from build123d import *

# Parameters (mm, degrees)
BOSS_EXTRUDE1_DEPTH     = 110
SKETCH2_R               = 8.1
CUT_EXTRUDE1_DEPTH      = 41
CUT_EXTRUDE2_DEPTH      = 74
CUT_EXTRUDE2_DEPTH_BACK = 41
SKETCH3_R               = 2.25
CUT_EXTRUDE3_DEPTH      = 21
SKETCH5_R               = 3.6
CUT_EXTRUDE4_DEPTH      = 17
SKETCH6_R               = 10
SKETCH6_R_2             = 2
CUT_EXTRUDE5_DEPTH      = 149
SKETCH7_R               = 1.5
CUT_EXTRUDE6_DEPTH      = 43


with BuildPart() as part:
    # Sketch1 → Boss-Extrude1 (new body)
    with BuildSketch(Plane.XY):
        with BuildLine():
            Line((0, 0), (40, 0))
            Line((40, 0), (20, -79.858784278))
            ThreePointArc((20, -79.858784278), (12.904134464, -90.766668728), (0.599169725, -95))
            Line((0.599169725, -95), (-73, -95))
            Line((-73, -95), (-73, -75))
            Line((-73, -75), (-20, -75))
            ThreePointArc((-20, -75), (-5.857864376, -69.142135624), (0, -55))
            Line((0, -55), (0, 0))
        make_face()
    extrude(amount=BOSS_EXTRUDE1_DEPTH)

    # Sketch2 → Cut-Extrude1 (cut, through all)
    with BuildSketch(Plane(origin=(0, -4.784896585, 0), x_dir=(0, 0, -1), z_dir=(1, 0, 0))):
        with Locations((-55, 4.784896585)):
            Circle(SKETCH2_R)
    extrude(amount=CUT_EXTRUDE1_DEPTH, mode=Mode.SUBTRACT)

    # Sketch4 → Cut-Extrude2 (cut, two sides)
    with BuildSketch(Plane.ZY) as cut_extrude2_sk:
        Polygon((33, 0), (0, -95), (0, 0), align=None)
        Polygon((77, 0), (110, -95), (110, 0), align=None)
    extrude(amount=CUT_EXTRUDE2_DEPTH, mode=Mode.SUBTRACT)
    extrude(cut_extrude2_sk.sketch, amount=-CUT_EXTRUDE2_DEPTH_BACK, mode=Mode.SUBTRACT)

    # Sketch3 → Cut-Extrude3 (cut, through all)
    with BuildSketch(Plane(origin=(0, -75, 0), x_dir=(1, 0, 0), z_dir=(0, 1, 0))):
        with Locations((-62.4, -12.5)):
            Circle(SKETCH3_R)
        with Locations((-62.4, -97.5)):
            Circle(SKETCH3_R)
        with Locations((-37.4, -12.5)):
            Circle(SKETCH3_R)
        with Locations((-37.4, -97.5)):
            Circle(SKETCH3_R)
    extrude(amount=-CUT_EXTRUDE3_DEPTH, mode=Mode.SUBTRACT)

    # Sketch5 → Cut-Extrude4 (cut)
    with BuildSketch(Plane(origin=(0, 0, 0), x_dir=(1, 0, 0), z_dir=(0, 1, 0))):
        with Locations((7, -40)):
            Circle(SKETCH5_R)
        with Locations((32, -40)):
            Circle(SKETCH5_R)
        with Locations((7, -70)):
            Circle(SKETCH5_R)
        with Locations((32, -70)):
            Circle(SKETCH5_R)
    extrude(amount=-CUT_EXTRUDE4_DEPTH, mode=Mode.SUBTRACT)

    # Sketch6 → Cut-Extrude5 (cut)
    with BuildSketch(Plane.ZY.offset(73)):
        with Locations((55, -95)):
            Circle(SKETCH6_R)
        with Locations((30, -85)):
            Circle(SKETCH6_R_2)
        with Locations((80, -85)):
            Circle(SKETCH6_R_2)
    extrude(amount=-CUT_EXTRUDE5_DEPTH, mode=Mode.SUBTRACT)

    # Sketch7 → Cut-Extrude6 (cut)
    with BuildSketch(Plane(origin=(37.639221534, -9.426444911, 0), x_dir=(0, 0, -1), z_dir=(0.970041514, -0.242939214, 0))):
        with Locations((-75, -22.607551707)):
            Circle(SKETCH7_R)
        with Locations((-35, -22.607551707)):
            Circle(SKETCH7_R)
    extrude(amount=-CUT_EXTRUDE6_DEPTH, mode=Mode.SUBTRACT)


solid = part.part
CAD build for the part. Positions are in the model's coordinates, mm. A direction names the side the tool comes from. Give positions to 0.01 mm unless a question says otherwise; leave off trailing zeros. Loops run counter-clockwise (first coordinate to the right, second up) from the corner with the lowest first, then second, coordinate; pieces in that order, holes last. Notation, with made-up numbers: M 79,-2 L 136,-2 A34 ccw 136,37 Z; hole C -30.75,33.5 d2. An arc over 180 degrees is marked long. Answer in a Markdown table with one row per item. Add a question column.
Item 1: Drop flat-ended pins along their axis: P1, Ø6, axis at x = -55, z = 86.5, coming from the +Y side; P2, Ø10, axis at y = -57.5, z = 14, coming from the +X side; P3, Ø6, axis at x = 32, z = 40, coming from the +Y side; P4, Ø7, axis at x = -37.4, z = 97.5, coming from the -Y side. Give the stop position or say it passes through.
Item 2: Band-saw the part on B-B on z = 30. Give the cut face in (x, y), then the cut area to 3 significant figures.
Item 3: Probe probe 1 along X at (y, z) = (-5, 70); probe 2 along Z at (x, y) = (-37.4, -82.5); probe 3 along Z at (x, y) = (-37.5, -80). List the from-to ranges inside material, lowest first.
Item 4: Band-saw the part on C-C on y = -14.5. Give the cut face in (x, z), then the cut area to 3 significant figures.
Item 5: Mould opens along Z. For faces 4 (the face through (-47, -75, 54)), 5 (the face through (7.82, -57.391, 96.936)), 6 (the face through (16.329, -26.35, 36.106)), 7 (the face through (-27.679, -83.314, 31.075)) say: +Z half, -Z half, draft (parallel to the pull), parting line (faces both ways), or undercut.
Item 6: Band-saw the part on A-A on x = -37.4. Give the cut face in (y, z).
Item 7: Band-saw the part on D-D on z = 70. Give the cut face in (x, y), then the cut area to 3 significant figures.
Item 8: Tool access for faces 1 (the face through (32, -17, 40)), 2 (the face through (0, -34, 54)), 3 (the face through (-36, -95, 22)): list every direction of +Z, -Z, +X, -X, +Y, -Y with a clear straight run to the whole face (end or side of a thin tool).
Reply:
| question | item | result |
|---|---|---|
| 1 | P1 | stops at y = -75 |
| 1 | P2 | stops at x = 26.84 |
| 1 | P3 | stops at y = -17 |
| 1 | P4 | stops at y = -95 |
| 2 | outline | M -73,-95 L 0.6,-95 A20 ccw 16.6,-87 L -73,-87 Z; M -73,-83 L 18.93,-83 A20 ccw 20,-79.86 L 37.84,-8.64 L 0,-8.64 L 0,-55 A20 cw -20,-75 L -73,-75 Z |
| 2 | area | 3,470 mm^2 |
| 3 | probe 1 | x = 0 to 3.4, 10.6 to 28.4, 35.6 to 38.75 |
| 3 | probe 2 | z = 4.34 to 10.25, 14.75 to 95.25, 99.75 to 105.66 |
| 3 | probe 3 | z = 5.21 to 10.25, 14.75 to 95.25, 99.75 to 104.79 |
| 4 | outline | M 0,27.96 L 36.37,27.96 L 36.37,82.04 L 0,82.04 Z; hole C 7,40 d7.2; hole C 7,70 d7.2; hole C 32,40 d7.2; hole C 32,70 d7.2 |
| 4 | area | 1,800 mm^2 |
| 5 | face 4 | draft |
| 5 | face 5 | +Z half |
| 5 | face 6 | undercut |
| 5 | face 7 | undercut |
| 6 | outline | M -95,0 L -75,6.95 L -75,10.25 L -95,10.25 Z; M -95,14.75 L -75,14.75 L -75,95.25 L -95,95.25 L -95,65 A10 cw -95,45 Z; M -95,99.75 L -75,99.75 L -75,103.05 L -95,110 Z; hole C -85,30 d4; hole C -85,80 d4 |
| 7 | outline | M -73,-95 L 0.6,-95 A20 ccw 20,-79.86 L 40,0 L 35.6,0 L 35.6,-17 L 28.4,-17 L 28.4,0 L 10.6,0 L 10.6,-17 L 3.4,-17 L 3.4,0 L 0,0 L 0,-55 A20 cw -20,-75 L -73,-75 Z |
| 7 | area | 3,920 mm^2 |
| 8 | face 1 | +Y |
| 8 | face 2 | +Z, -Z, -X, +Y |
| 8 | face 3 | +Z, -Z, +X, -X, -Y |
